Could you check a few things on this model? Use its own coordinates, in mm. A direction names the side the tool comes from. Round coordinates to 2 decimals unless told otherwise and drop trailing zeros. Loops run counter-clockwise (first coordinate to the right, second up) from the corner with the lowest first, then second, coordinate; pieces in that order, holes last. Notation, with made-up numbers: (26, 81.5) - (79, 81.5) arc R24 cw to (79, 102.5) - close; hole circle Ø6 at (87.25, 34.5). An arc over 180 degrees is marked (long way). Answer as CSV lines item,"result". Start each with the question number.
1) Suppose I cut it at A-A, the plane z = 192.5. Write out the boundary of the cut face in (x, y), then the cut area to 3 significant figures.
2) Which directions (+Z, -Z, +X, -X, +Y, -Y) give clear straight access to the entire face, cutting with the end or side of a thin tool? Please do faces 1 (the face through (8, 2, 115)), 2 (the face through (71, -5, 212.1)).
3) Suppose I cut it at C-C, the plane y = -4. Write out the boundary of the cut face in (x, z).
4) Suppose I cut it at B-B, the plane x = 46. Write out the boundary of the cut face in (y, z), then the cut area to 3 significant figures.
5) We'd pull the mould along X, two halves only. Please class faces 3 (the face through (143.8, -4, 106)), 4 (the face through (71, -4, 214.1)), 5 (the face through (0, -4, 106)), 6 (the face through (141.8, -5, 109)): pulls with the +X half, pulls with the -X half, needs draft (parallel to the pull), parting line crosses it, or undercut.
6) Please list where these lines run through material, in increasing order: line 1 along Z through (x, y) = (36.5, -0.5); line 2 along X through (y, z) = (-2, 175); line 3 along Z through (x, y) = (78, 0.25).
```python
from build123d import *

# Parameters (mm, degrees)
F0_W     = 143.8
F0_H     = 214.1
F1_DEPTH = 10
F2_DEPTH = 2


with BuildPart() as f1:
    # F0 (on Front) → F1 (new body)
    with BuildSketch(Plane.XZ):
        with Locations((71.9, 107.05)):
            Rectangle(F0_W, F0_H)
        Polygon((2, 149.1), (2, 212.1), (78.8, 212.1), (141.8, 212.1), (141.8, 149.1), (141.8, 2), (78.8, 2), (2, 2), align=None, mode=Mode.SUBTRACT)
    extrude(amount=F1_DEPTH)

    # F0 (on Front) → F2 (join)
    with BuildSketch(Plane.XZ):
        with Locations((71.9, 107.05)):
            Rectangle(F0_W, F0_H)
        Polygon((2, 149.1), (2, 212.1), (78.8, 212.1), (141.8, 212.1), (141.8, 149.1), (141.8, 2), (78.8, 2), (2, 2), align=None, mode=Mode.SUBTRACT)
        Polygon((78.8, 212.1), (2, 212.1), (2, 149.1), (12, 149.1), (12, 202.1), (78.8, 202.1), align=None)
        Polygon((141.8, 212.1), (78.8, 212.1), (78.8, 202.1), (131.8, 202.1), (131.8, 149.1), (141.8, 149.1), align=None)
        Polygon((12, 149.1), (2, 149.1), (2, 2), (78.8, 2), (78.8, 12), (12, 12), align=None)
        Polygon((141.8, 2), (141.8, 149.1), (131.8, 149.1), (131.8, 12), (78.8, 12), (78.8, 2), align=None)
    extrude(amount=-F2_DEPTH)


solid = f1.part
```
Filled sheet:
1,outline,"(0, -10) - (2, -10) - (2, 0) - (12, 0) - (12, 2) - (0, 2) - close; (131.8, 0) - (141.8, 0) - (141.8, -10) - (143.8, -10) - (143.8, 2) - (131.8, 2) - close"
1,area,"88.0 mm²"
2,face 1,"+Z, -Z, +X, -X, +Y"
2,face 2,"-Y"
3,outline,"(0, 0) - (143.8, 0) - (143.8, 214.1) - (0, 214.1) - close; hole (2, 2) - (141.8, 2) - (141.8, 212.1) - (2, 212.1) - close"
4,outline,"(-10, 0) - (2, 0) - (2, 12) - (0, 12) - (0, 2) - (-10, 2) - close; (-10, 212.1) - (0, 212.1) - (0, 202.1) - (2, 202.1) - (2, 214.1) - (-10, 214.1) - close"
4,area,"88.0 mm²"
5,face 3,"pulls with the +X half"
5,face 4,"needs draft"
5,face 5,"pulls with the -X half"
5,face 6,"undercut"
6,line 1,"0 to 2, 212.1 to 214.1"
6,line 2,"0 to 2, 141.8 to 143.8"
6,line 3,"0 to 12, 202.1 to 214.1"
